CAD build for the part. Positions are in the model's coordinates, mm. Give positions to 0.01 mm unless a question says otherwise; leave off trailing zeros. Loops run counter-clockwise (first coordinate to the right, second up) from the corner with the lowest first, then second, coordinate; pieces in that order, holes last.
```python
from build123d import *

# Parameters (mm, degrees)
ESQUISSE2_R   = 3
ESQUISSE2_R_2 = 2


with BuildPart() as part:
    # Balayage1: sweep along a curve in space
    with BuildLine() as balayage1_path:
        Line((0, 0, 0), (0, 150, 0))
        ThreePointArc((0, 150, 0), (0, 164.142135624, 5.857864376), (0, 170, 20))
        Line((0, 170, 20), (0, 170, 60))
        ThreePointArc((0, 170, 60), (-5.857864376, 170, 74.142135624), (-20, 170, 80))
        Line((-20, 170, 80), (-200, 170, 80))
    # Esquisse2 → Balayage1 (sweep)
    with BuildSketch(Plane(origin=(0, 0, 0), x_dir=(1, 0, 0), z_dir=(0, 1, 0))):
        Circle(ESQUISSE2_R)
        Circle(ESQUISSE2_R_2, mode=Mode.SUBTRACT)
    sweep(path=balayage1_path.line)


solid = part.part
```
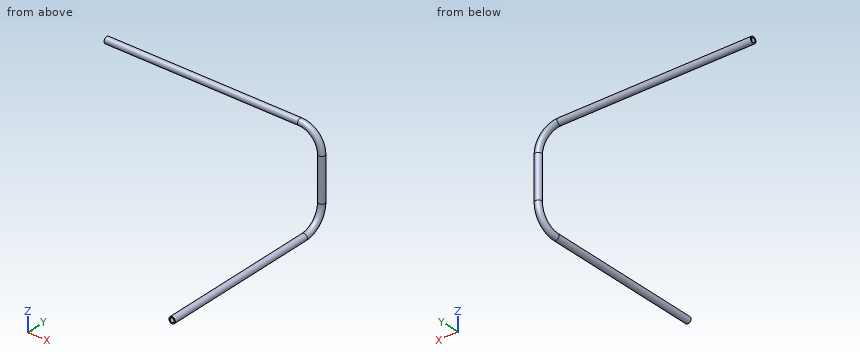
1. Saw through at B-B, the plane y = 51. List the corners of the cut face in (x, z).
Responses:
outline: circle Ø6 at (0, 0); hole circle Ø4 at (0, 0)
2. Drop flat-ended pins along their axis: pin 1 (4.5 mm diameter, centred on x = 0, z = 0, fed in from +Y); pin 2 (2.5 mm diameter, centred on x = 0, y = 170, fed in from -Z); pin 3 (2.5 mm diameter, centred on y = 170, z = 80, fed in from +X). Give the stop position or say it passes through.
Responses:
pin 1: stops at y = 164.63
pin 2: stops at z = 6.68
pin 3: stops at x = -6.68
3. Saw through at A-A, the plane x = -173. List the corners of the cut face in (y, z), and give its area (3 significant figures).
Responses:
outline: circle Ø6 at (170, 80); hole circle Ø4 at (170, 80)
area: 15.7 mm2
4. Probe line 1 along Y through (x, z) = (0, 39); line 2 along Z through (x, y) = (-83, 170); line 3 along Z through (x, y) = (0, 35). List the from-to ranges inside material, lowest first.
Responses:
line 1: y = 167 to 168, 172 to 173
line 2: z = 77 to 78, 82 to 83
line 3: z = -3 to -2, 2 to 3
